Verification items for the finished model (mm, model axes). Give positions to 0.01 mm unless a question says otherwise; leave off trailing zeros. Loops run counter-clockwise (first coordinate to the right, second up) from the corner with the lowest first, then second, coordinate; pieces in that order, holes last. Notation, with made-up numbers: (52, 83.25) - (73, 83.25) arc R22 cw to (73, 103.25) - close; hole circle Ø1 at (83.25, 32.5). An arc over 180 degrees is marked (long way). Answer in a Markdown table with one row per item.
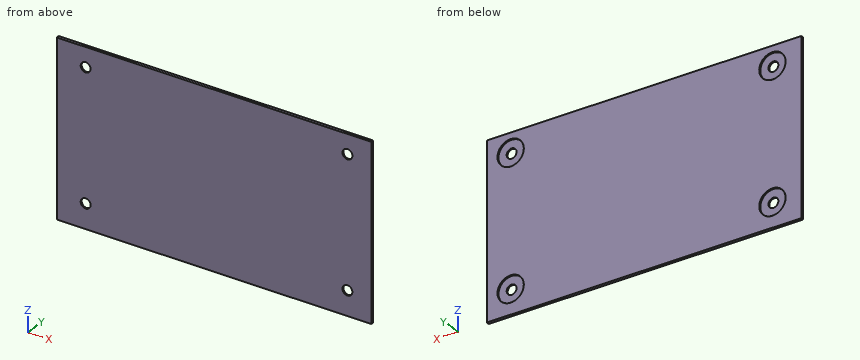
```python
from build123d import *

# Parameters (mm, degrees)
SKETCH_2_W                  = 108
SKETCH_2_H                  = 60
EXTRUDE_1_DEPTH             = 1
HOLE_WIZARD_M3_1_AT_2_COUNT = 2
HOLE_WIZARD_M3_1_AT_2_PITCH = 89.888096236
HOLE_WIZARD_M3_1_AT_3_COUNT = 2
HOLE_WIZARD_M3_1_AT_3_PITCH = 44.863801861
HOLE_WIZARD_M3_1_AT_4_COUNT = 2
HOLE_WIZARD_M3_1_AT_4_PITCH = 100.462085198


with BuildPart() as part:
    # 草图2 → 凸台-拉伸1 (new body)
    with BuildSketch(Plane(origin=(0, 0, 0), x_dir=(1, 0, 0), z_dir=(0, 1, 0))):
        Rectangle(SKETCH_2_W, SKETCH_2_H)
    extrude(amount=EXTRUDE_1_DEPTH)

    # 草图4 → M3 六角头螺栓的柱形沉头孔1 (revolve, cut)
    with BuildSketch(Plane(origin=(-44.084962343, 1, -21.539091549), x_dir=(0, 0, 1), z_dir=(1, 0, 0))):
        Polygon((0, 0), (0, 1), (1.7, 1), (1.7, 0.5), (4.5, 0.5), (4.5, 0.025), (4.525, 0), align=None)
    hole_wizard_m3_1 = revolve(axis=Axis((-44.084962343, 7.35, -21.539091549), (0, -1, 0)), mode=Mode.SUBTRACT)

    # M3 六角头螺栓的柱形沉头孔1 at 2: M3 六角头螺栓的柱形沉头孔1 ×2
    with Locations(*[(i * HOLE_WIZARD_M3_1_AT_2_PITCH, 0, 0) for i in range(1, HOLE_WIZARD_M3_1_AT_2_COUNT)]):
        add(hole_wizard_m3_1, mode=Mode.SUBTRACT)

    # M3 六角头螺栓的柱形沉头孔1 at 3: M3 六角头螺栓的柱形沉头孔1 ×2
    with Locations(*[(0, 0, i * HOLE_WIZARD_M3_1_AT_3_PITCH) for i in range(1, HOLE_WIZARD_M3_1_AT_3_COUNT)]):
        add(hole_wizard_m3_1, mode=Mode.SUBTRACT)

    # M3 六角头螺栓的柱形沉头孔1 at 4: M3 六角头螺栓的柱形沉头孔1 ×2
    with Locations(*[Vector(0.894746471, 0, 0.446574464) * (i * HOLE_WIZARD_M3_1_AT_4_PITCH) for i in range(1, HOLE_WIZARD_M3_1_AT_4_COUNT)]):
        add(hole_wizard_m3_1, mode=Mode.SUBTRACT)


solid = part.part
```
Q1. Go/stop test with flat-tipped pins: P1, Ø7, axis at x = -44, z = -22.5, coming from the +Y side; P2, Ø2, axis at x = 45.8, z = 23.32, coming from the +Y side. Record where each tip stops, or that it passes through.
Completed:
| item | result |
|---|---|
| P1 | y = 0.5 |
| P2 | through |
Q2. Sectioned sample at A-A (y = 0.75). Record the cut outline in (x, z).
Completed:
| item | result |
|---|---|
| outline | (-54, -30) - (54, -30) - (54, 30) - (-54, 30) - close; hole circle Ø9 at (-44.08, -21.54); hole circle Ø9 at (-44.08, 23.32); hole circle Ø9 at (45.8, -21.54); hole circle Ø9 at (45.8, 23.32) |
Q3. Thickness scan on line 1 (X direction, y = 0.45, z = 23.5); line 2 (X direction, y = 0.6, z = 25); line 3 (Z direction, x = -45.5, y = 0.25). Record the ranges inside material, lowest first.
Completed:
| item | result |
|---|---|
| line 1 | -54 to -45.78, -42.39 to 44.11, 47.49 to 54 |
| line 2 | -54 to -48.26, -39.91 to 41.63, 49.98 to 54 |
| line 3 | -30 to -22.48, -20.6 to 22.38, 24.27 to 30 |
